The listing builds one solid part. Answer for the finished solid, in the listing's coordinates (mm). A direction names the side the tool comes from. Coordinates: 2 decimals unless noted, no trailing zeros. Loops run counter-clockwise (first coordinate to the right, second up) from the corner with the lowest first, then second, coordinate; pieces in that order, holes last. Notation, with made-up numbers: M -4.75,18.5 L 42.25,18.5 A25 cw 42.25,39.5 Z; hole C 79,64 d5. An arc over 180 degrees is marked long. Return JSON: item names as keys, results as strings. Group by question number.
1. Section B-B (z = 1.95) is taken. Write down the section's boundary in (x, y) (3 decimals), then the cut area to 3 significant figures.
2. Section D-D (z = 3.65) is taken. Write down the section's boundary in (x, y) (3 decimals).
3. The mould has two halves that part along Y. Classify faces 3 (the face through (-6.245, -39.924, 2.958)), 4 (the face through (0, -24, 3.175)), 5 (the face through (-7.43, -49.4, 3.04)): pulls with the +Y half, pulls with the -Y half, needs draft (parallel to the pull), parting line crosses it, or undercut.
4. Section A-A (x = -5) is taken. Write down the section's boundary in (y, z) (3 decimals), then the cut area to 3 significant figures.
5. Section C-C (y = -24.85) is taken. Write down the section's boundary in (x, z) (3 decimals).
6. Given P1, Ø4, axis at x = 5, y = -24.85, coming from the +Z side (3 decimals), flat-ended and moving along its own axis, determine where the tip first touches the part or whether it passes through.
7. Which of the six approach directions +Z, -Z, +X, -X, +Y, -Y give full straight-line access (tool end or side, diameter ignored) to faces 1 (the face through (0, -27.4, 5)), 2 (the face through (0, -50, 3))?
8. Straight lines are drawn through the part: L1, parallel to Y at x = -5, z = 0.9; L2, parallel to Y at x = -0.5, z = 4.75; L3, parallel to Y at x = -7, z = 4.7. For each, find the intervals that lie inside material, in ascending order. Write a range as from..to.
```python
from build123d import *

# Parameters (mm, degrees)
SKETCH1_W               = 16
SKETCH1_H               = 30
SKETCH1_R               = 1.6
BOSS_EXTRUDE1_DEPTH     = 3.175
SKETCH3_W               = 16
SKETCH3_H               = 22.6
BOSS_EXTRUDE2_DEPTH     = 6
FILLET1_R               = 2
CUT_EXTRUDE1_DEPTH      = 51.735398146
CUT_EXTRUDE1_DEPTH_BACK = 51.735398146


with BuildPart() as part:
    # Sketch1 → Boss-Extrude1 (new body)
    with BuildSketch(Plane.XY):
        with Locations((0, -35)):
            Rectangle(SKETCH1_W, SKETCH1_H)
        with Locations((5, -24.85)):
            Circle(SKETCH1_R, mode=Mode.SUBTRACT)
        with Locations((-5, -24.85)):
            Circle(SKETCH1_R, mode=Mode.SUBTRACT)
    extrude(amount=BOSS_EXTRUDE1_DEPTH)

    # Sketch3 → Boss-Extrude2 (add)
    with BuildSketch(Plane(origin=(0, 0, 0), x_dir=(-1, 0, 0), z_dir=(0, 0, -1))):
        with Locations((0, -38.7)):
            Rectangle(SKETCH3_W, SKETCH3_H)
    extrude(amount=-BOSS_EXTRUDE2_DEPTH)

    # Fillet1
    fillet1_edges = [part.edges().sort_by_distance(p)[0] for p in [
        (8, -50, 3),
        (-8, -50, 3),
    ]]
    fillet(fillet1_edges, radius=FILLET1_R)

    # Sketch4 → Cut-Extrude1 (cut, two sides: drawn at the far end of the back side and taken through both)
    with BuildSketch(Plane.XY.offset(3.175).offset(-CUT_EXTRUDE1_DEPTH_BACK)):
        with BuildLine():
            Line((-8, -45), (-8, -35))
            ThreePointArc((-8, -35), (-6.244997998, -40), (-8, -45))
        make_face()
    extrude(amount=CUT_EXTRUDE1_DEPTH + CUT_EXTRUDE1_DEPTH_BACK, mode=Mode.SUBTRACT)


solid = part.part
```
Worked out:
{
 "1": {"outline": "M -8,-48 A2 ccw -6,-50 L 6,-50 A2 ccw 8,-48 L 8,-20 L -8,-20 L -8,-35 A8 cw -8,-45 Z; hole C -5,-24.85 d3.2; hole C 5,-24.85 d3.2", "area": "450 mm^2"},
 "2": {"outline": "M -8,-48 A2 ccw -6,-50 L 6,-50 A2 ccw 8,-48 L 8,-27.4 L -8,-27.4 L -8,-35 A8 cw -8,-45 Z"},
 "3": {"face 3": "undercut", "face 4": "needs draft", "face 5": "pulls with the -Y half"},
 "4": {"outline": "M -50,0 L -26.45,0 L -26.45,3.175 L -27.4,3.175 L -27.4,6 L -50,6 Z; M -23.25,0 L -20,0 L -20,3.175 L -23.25,3.175 Z", "area": "149 mm^2"},
 "5": {"outline": "M -8,0 L -6.6,0 L -6.6,3.175 L -8,3.175 Z; M -3.4,0 L 3.4,0 L 3.4,3.175 L -3.4,3.175 Z; M 6.6,0 L 8,0 L 8,3.175 L 6.6,3.175 Z"},
 "6": {"P1": "z = 3.175"},
 "7": {"face 1": "+Z, +X, -X, +Y", "face 2": "+Z, -Z, +X, -X, -Y"},
 "8": {"L1": "-50..-26.45, -23.25..-20", "L2": "-50..-27.4", "L3": "-49.73..-43.39, -36.61..-27.4"}
}
